Could you check a few things on this model? Use its own coordinates, in mm. Face numbers are marked on the shaded views. A direction names the side the tool comes from. Give positions to 0.01 mm unless a question says otherwise; leave off trailing zeros. Write each loop counter-clockwise with the first axis right and the second up, starting at its lowest first coordinate (ties: lowest second). Pieces come first, ordered by that corner, then holes. Notation, with made-up numbers: M -34,-5 L -14,-5 A23 ccw -14,3 Z; hole C -17,85 d11. An arc over 180 degrees is marked long. Write each question's results on one line, items separated by ' | '. Start each with the question number.
from build123d import *

# Parameters (mm, degrees)
SKETCH_1_R               = 7
SKETCH_1_R_2             = 3
EXTRUDE_1_DEPTH          = 8.5
SKETCH_2_R               = 6
SKETCH_2_R_2             = 1.75
EXTRUDE_2_DEPTH          = 10.5
FILLET_1_R               = 1
SKETCH_3_R               = 1.5
CUT_EXTRUDE_1_DEPTH      = 14.5
CUT_EXTRUDE_2_DEPTH      = 6.5
CUT_EXTRUDE_2_DEPTH_BACK = 6.5
SKETCH_4_R               = 1.5


with BuildPart() as part:
    # Sketch 1 → Extrude 1 (new body)
    with BuildSketch(Plane(origin=(0, 0, 0), x_dir=(1, 0, 0), z_dir=(0, 1, 0))):
        with Locations(Location((-14.312366838, 6.407280503, 0), (0, 0, 270))):
            Circle(SKETCH_1_R)
        with Locations(Location((-14.312366838, 6.407280503, 0), (0, 0, 270))):
            Circle(SKETCH_1_R_2, mode=Mode.SUBTRACT)
    extrude(amount=EXTRUDE_1_DEPTH)

    # Sketch 2 → Extrude 2 (add)
    with BuildSketch(Plane(origin=(0, 8.5, 0), x_dir=(1, 0, 0), z_dir=(0, 1, 0))):
        with Locations(Location((-14.312366838, 6.407280503, 0), (0, 0, 90))):
            Circle(SKETCH_2_R)
        with Locations(Location((-14.312366838, 6.407280503, 0), (0, 0, 90))):
            Circle(SKETCH_2_R_2, mode=Mode.SUBTRACT)
    extrude(amount=EXTRUDE_2_DEPTH)

    # Fillet 1
    fillet_1_edges = [part.edges().sort_by_distance(p)[0] for p in [
        (-14.312366838, 19, -0.407280503),
        (-14.312366838, 0, -13.407280503),
    ]]
    fillet(fillet_1_edges, radius=FILLET_1_R)

    # Sketch 3 → Cut-Extrude 1 (cut)
    with BuildSketch(Plane(origin=(0, 0, 0), x_dir=(0, 0, -1), z_dir=(1, 0, 0))):
        with Locations((6.442812973, 3.5)):
            Circle(SKETCH_3_R)
    extrude(amount=-CUT_EXTRUDE_1_DEPTH, mode=Mode.SUBTRACT)

    # Sketch 4 → Cut-Extrude 2 (cut, two sides: drawn at the far end of the back side and taken through both)
    with BuildSketch(Plane.XY.offset(-CUT_EXTRUDE_2_DEPTH_BACK)):
        with Locations(Location((-14.374144883, 3.5, 0), (0, 0, 180))):
            Circle(SKETCH_4_R)
    extrude(amount=CUT_EXTRUDE_2_DEPTH + CUT_EXTRUDE_2_DEPTH_BACK, mode=Mode.SUBTRACT)


solid = part.part
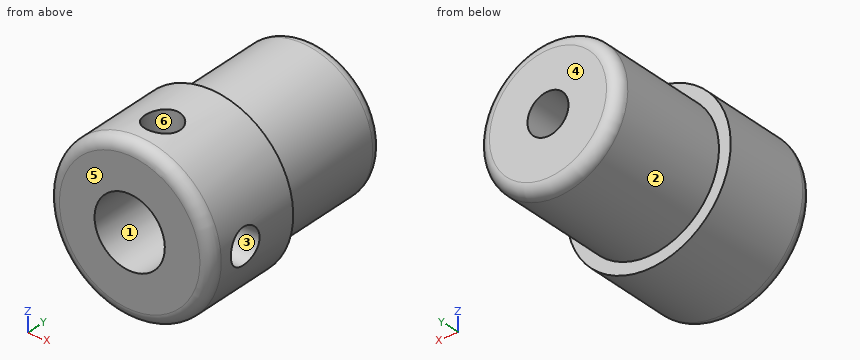
Q1. For the marked faces 1, 2 and 3, which set-ups out of +Z, -Z, +X, -X, +Y, -Y let a thin tool reach every point of the face, with its end or its side?
Q2. If we mould it in two halves opening along Y, with no side actions, what happens to the marked faces 4, 5 and 6? For each: pulls with the +Y half, pulls with the -Y half, needs draft (parallel to the pull), parting line crosses it, or undercut.
Q3. I'm going to push flat-ended pins straight in: P1, Ø6, axis at x = -9.5, z = -4.5, coming from the -Y side; P2, Ø3, axis at x = -10, y = 12.5, coming from the -Z side; P3, Ø4, axis at x = -10.5, y = 4, coming from the -Z side; P4, Ø1.5, axis at x = -12.5, y = 4.5, coming from the +Z side. Where does each tip first touch, or does it pass through?
Q4. If we section it at A-A (y = 3.5): Please give me the cut outline in (x, z).
Q5. Please list where these lines run through material, in increasing order: line 1 (Z direction, x = -14.5, y = 1.5); line 2 (Y direction, x = -11, z = -6.75); line 3 (Y direction, x = -8.75, z = -7.5). Write a range as [from, to].
Q6. If we section it at D-D (y = 16): Please give me the cut outline in (x, z), plus the area to 3 significant figures.
Q7. If we section it at B-B (z = -7): Count the separate pieces of the cut face and the enclosed holes in it, plus the area to 3 significant figures.
Determined:
1) face 1: -Y | face 2: +Y | face 3: +X
2) face 4: pulls with the +Y half | face 5: pulls with the -Y half | face 6: undercut
3) P1: stops at y = 0 | P2: stops at z = -11.71 | P3: stops at z = -13.17 | P4: stops at z = 0.51
4) outline: M -15.87,-3.85 L -15.87,0.42 A7 ccw long -7.48,-7.94 L -11.74,-7.94 A3 cw long Z; M -12.87,-3.77 A3 cw -11.69,-4.94 L -7.47,-4.94 A7 ccw -12.87,0.44 Z
5) line 1: z = [-13.4, -9.4], [-3.41, 0.59] | line 2: y = [0, 2.03], [4.97, 19] | line 3: y = [0, 2.44], [4.56, 18.74]
6) outline: C -14.31,-6.41 d12; hole C -14.31,-6.41 d3.5 | area: 103 mm²
7) separate pieces: 3 | enclosed holes: 0 | area: 147 mm²
